```python
from build123d import *

# Parameters (mm, degrees)
F0_W     = 5
F0_H     = 15
F2_W     = 4.3588989435
F2_H     = 9
F3_DEPTH = 9
F4_R     = 3.1991269496
F5_DEPTH = 5
F6_W     = 4.3588989435
F6_H     = 9
F7_DEPTH = 9
F8_R     = 3.25
F9_DEPTH = 5


with BuildPart() as f1:
    # F0 (on Top) → F1 (revolve)
    with BuildSketch(Plane.XY):
        with Locations((-2.5, 7.5)):
            Rectangle(F0_W, F0_H)
    revolve(axis=Axis((0, 7.5, 0), (0, 1, 0)))

    # F2 (on face) → F3 (join)
    with BuildSketch(Plane.XZ):
        Rectangle(F2_W, F2_H)
    extrude(amount=F3_DEPTH)

    # F4 (on face) → F5 (cut)
    with BuildSketch(Plane(origin=(-2.1794494718, 0, 0), x_dir=(0, -1, 0), z_dir=(-1, 0, 0))):
        with Locations((4.5, 0)):
            Circle(F4_R)
    extrude(amount=-F5_DEPTH, mode=Mode.SUBTRACT)

    # F6 (on face) → F7 (join)
    with BuildSketch(Plane(origin=(0, 15, 0), x_dir=(-1, 0, 0), z_dir=(0, 1, 0))):
        Rectangle(F6_W, F6_H)
    extrude(amount=F7_DEPTH)

    # F8 (on face) → F9 (cut)
    with BuildSketch(Plane(origin=(-2.1794494718, 0, 0), x_dir=(0, -1, 0), z_dir=(-1, 0, 0))):
        with Locations((-19.5, 0)):
            Circle(F8_R)
    extrude(amount=-F9_DEPTH, mode=Mode.SUBTRACT)


solid = f1.part
```
Work out the finished part from the listing and answer in its coordinate system (mm). A direction names the side the tool comes from. Coordinates: 2 decimals unless noted, no trailing zeros. Loops run counter-clockwise (first coordinate to the right, second up) from the corner with the lowest first, then second, coordinate; pieces in that order, holes last. Notation, with made-up numbers: (56.5, 6.5) -> (95.5, 6.5) arc R13 cw to (95.5, 23.5) -> close; hole circle Ø10 at (26.25, -29.5). An arc over 180 degrees is marked (long way). Answer as CSV lines item,"result".
Q1. The part is cut by section C-C on z = 0. Write down the section's boundary in (x, y).
Findings:
outline,"(-5, 0) -> (-2.18, 0) -> (-2.18, -1.3) -> (2.18, -1.3) -> (2.18, 0) -> (5, 0) -> (5, 15) -> (2.18, 15) -> (2.18, 16.25) -> (-2.18, 16.25) -> (-2.18, 15) -> (-5, 15) -> close; (-2.18, -9) -> (2.18, -9) -> (2.18, -7.7) -> (-2.18, -7.7) -> close; (-2.18, 22.75) -> (2.18, 22.75) -> (2.18, 24) -> (-2.18, 24) -> close"
Q2. A tool of negligible diameter and unlimited length cuts with its end or side. For faces 4 (the face through (0, 19, 4.5)), 5 (the face through (0, -4, 4.5)), 6 (the face through (2.179, -3, -3)), 7 (the face through (2.179, 22.4, -2.1)), 8 (the face through (-3, 0, 0)), from which of +Z, -Z, +X, -X, +Y, -Y can it reach the whole face along a straight path? Write none if from no direction.
Findings:
face 4,"+Z, +X, -X, +Y"
face 5,"+Z, +X, -X, -Y"
face 6,"+Z, -Z, +X, -Y"
face 7,"+Z, -Z, +X, +Y"
face 8,"+Z, -Z, -X, -Y"
Q3. Each of these flat-tipped pins is pushed along its axis until it touches: pin 1 (3 mm diameter, centred on x = -0.5, y = -3, fed in from -Z); pin 2 (1.5 mm diameter, centred on x = -3.5, y = 5, fed in from +Z); pin 3 (3 mm diameter, centred on x = 4, z = 0, fed in from +Y); pin 4 (6 mm diameter, centred on x = 3, z = -0.5, fed in from +Y). Where does it stop, or does it pass through?
Findings:
pin 1,"stops at z = -4.5"
pin 2,"stops at z = 4.18"
pin 3,"stops at y = 15"
pin 4,"stops at y = 24"
Q4. The part is cut by section A-A on y = -4.5. Write down the section's boundary in (x, z), and give its area (3 significant figures).
Findings:
outline,"(-2.18, -4.5) -> (2.18, -4.5) -> (2.18, -3.2) -> (-2.18, -3.2) -> close; (-2.18, 3.2) -> (2.18, 3.2) -> (2.18, 4.5) -> (-2.18, 4.5) -> close"
area,"11.3 mm²"
Q5. The part is cut by section D-D on y = 19.5. Write down the section's boundary in (x, z).
Findings:
outline,"(-2.18, -4.5) -> (2.18, -4.5) -> (2.18, -3.25) -> (-2.18, -3.25) -> close; (-2.18, 3.25) -> (2.18, 3.25) -> (2.18, 4.5) -> (-2.18, 4.5) -> close"
Q6. For a pull along Z with two mould halves and no side action, classify faces 1 (the face through (-0.031, 22.747, 0.143)), 2 (the face through (0, -4, -4.5)), 3 (the face through (3, 15, 0)) as +Z half, -Z half, draft (parallel to the pull), parting line (faces both ways), or undercut.
Findings:
face 1,"undercut"
face 2,"-Z half"
face 3,"draft"
Q7. Find the intervals of material crossed by probe 1 along Y at (x, z) = (2, -0.5); probe 2 along X at (y, z) = (18, -4); probe 3 along Y at (x, z) = (-1, -2), in increasing order.
Findings:
probe 1,"y = -9 to -7.66, -1.34 to 16.29, 22.71 to 24"
probe 2,"x = -2.18 to 2.18"
probe 3,"y = -9 to -7, -2 to 16.94, 22.06 to 24"
Q8. The part is cut by section B-B on x = 0. Write down the section's boundary in (y, z), and give its area (3 significant figures).
Findings:
outline,"(-9, -4.5) -> (0, -4.5) -> (0, -5) -> (15, -5) -> (15, -4.5) -> (24, -4.5) -> (24, 4.5) -> (15, 4.5) -> (15, 5) -> (0, 5) -> (0, 4.5) -> (-9, 4.5) -> close; hole circle Ø6.4 at (-4.5, 0); hole circle Ø6.5 at (19.5, 0)"
area,"247 mm²"
